Part model, mm, in its own coordinate system. A direction names the side the tool comes from. Round coordinates to 2 decimals unless told otherwise and drop trailing zeros. Order: outer loops, then holes, each group sorted by start corner. A loop starts at its lowest first (then second) coordinate and runs counter-clockwise, first axis right, second up. Notation, with made-up numbers: (80.25, 87.5) - (101.25, 87.5) arc R25 cw to (101.25, 105.5) - close; hole circle Ø1 at (7.5, 45). An arc over 180 degrees is marked (long way). Return JSON: item names as keys, results as strings. Group by question number.
Item 1: Saw through at B-B on z = 6. State how many separate pieces and enclosed holes the cut face has, and give its area (3 significant figures).
Item 2: Saw through at A-A on x = 10. List the corners of the cut face in (y, z), and give its area (3 significant figures).
Item 3: Drop flat-ended pins along their axis: pin 1 (3 mm diameter, centred on x = 46.25, z = 6, fed in from -Y); pin 2 (6 mm diameter, centred on x = 23, z = 3, fed in from +Y). Give the stop position or say it passes through.
Item 4: Saw through at C-C on y = 39. List the corners of the cut face in (x, z), and give its area (3 significant figures).
Item 5: Saw through at D-D on z = 10.25. List the corners of the cut face in (x, y), and give its area (3 significant figures).
Item 6: Probe probe 1 along X at (y, z) = (2.55, 6); probe 2 along X at (y, z) = (25.5, 9); probe 3 along Y at (x, z) = (57.6, 6). List the from-to ranges inside material, lowest first.
Item 7: Two-plate mould, pull along Y, no slides. Class faces 6 (the face through (32, 0, 6)), 7 (the face through (59.4, 54, 6)), 8 (the face through (32, 3, 0)), 9 (the face through (60, 59, 6)): released by +Y, released by -Y, zero draft, split by the parting line, or undercut.
Item 8: Tool access for faces 1 (the face through (58.18, 51.46, 6.56)), 2 (the face through (19.584, 1.726, 6.241)), 3 (the face through (64, 29, 6)), 4 (the face through (55, 47, 6)), 5 (the face through (9, 45, 6)): list every direction of +Z, -Z, +X, -X, +Y, -Y with a clear straight run to the whole face (end or side of a thin tool).
```python
from build123d import *

# Parameters (mm, degrees)
SKETCH1_W           = 64
SKETCH1_H           = 59
SKETCH1_W_2         = 50
SKETCH1_H_2         = 52
BOSS_EXTRUDE1_DEPTH = 12
SKETCH2_R           = 1.85
CUT_EXTRUDE1_DEPTH  = 10
SKETCH3_R           = 1.85
CUT_EXTRUDE2_DEPTH  = 10
SKETCH4_W           = 50
SKETCH4_H           = 12
SKETCH4_R           = 1.85
CUT_EXTRUDE4_DEPTH  = 10
SKETCH6_R           = 2.6
CUT_EXTRUDE5_DEPTH  = 2.4
SKETCH7_W           = 12
SKETCH7_H           = 2
BOSS_EXTRUDE2_DEPTH = 4


with BuildPart() as part:
    # Sketch1 → Boss-Extrude1 (new body)
    with BuildSketch(Plane.XY):
        with Locations((32, 29.5)):
            Rectangle(SKETCH1_W, SKETCH1_H)
        with Locations((32, 29.5)):
            Rectangle(SKETCH1_W_2, SKETCH1_H_2, mode=Mode.SUBTRACT)
    extrude(amount=BOSS_EXTRUDE1_DEPTH)

    # Sketch2 → Cut-Extrude1 (cut)
    with BuildSketch(Plane(origin=(0, 59, 0), x_dir=(1, 0, 0), z_dir=(0, 1, 0))):
        with Locations(Location((18, -9.7, 0), (0, 0, 180))):
            Circle(SKETCH2_R)
        with Locations(Location((46, -9.7, 0), (0, 0, 180))):
            Circle(SKETCH2_R)
        with Locations(Location((32, -9.7, 0), (0, 0, 180))):
            Circle(SKETCH2_R)
    extrude(amount=-CUT_EXTRUDE1_DEPTH, mode=Mode.SUBTRACT)

    # Sketch3 → Cut-Extrude2 (cut)
    with BuildSketch(Plane.XZ):
        with Locations(Location((17.75, 6, 0), (0, 0, 270))):
            Circle(SKETCH3_R)
        with Locations(Location((46.25, 6, 0), (0, 0, 180))):
            Circle(SKETCH3_R)
    extrude(amount=-CUT_EXTRUDE2_DEPTH, mode=Mode.SUBTRACT)

    # Sketch4 → Cut-Extrude4 (cut)
    with BuildSketch(Plane(origin=(0, 59, 0), x_dir=(1, 0, 0), z_dir=(0, 1, 0))):
        with Locations((32, -6)):
            Rectangle(SKETCH4_W, SKETCH4_H)
        with Locations((18, -9.7)):
            Circle(SKETCH4_R, mode=Mode.SUBTRACT)
        with Locations((32, -9.7)):
            Circle(SKETCH4_R, mode=Mode.SUBTRACT)
        with Locations((46, -9.7)):
            Circle(SKETCH4_R, mode=Mode.SUBTRACT)
    extrude(amount=-CUT_EXTRUDE4_DEPTH, mode=Mode.SUBTRACT)

    # Sketch6 → Cut-Extrude5 (cut)
    with BuildSketch(Plane(origin=(7, 0, 0), x_dir=(0, 0, -1), z_dir=(1, 0, 0))):
        with Locations((-6, 54)):
            Circle(SKETCH6_R)
    cut_extrude5 = extrude(amount=-CUT_EXTRUDE5_DEPTH, mode=Mode.SUBTRACT)

    # Mirror1: Cut-Extrude5 across plane
    add(cut_extrude5.mirror(Plane.ZY.offset(-32)), mode=Mode.SUBTRACT)

    # Sketch7 → Boss-Extrude2 (add)
    with BuildSketch(Plane.ZY.offset(-57)):
        with Locations((6, 46)):
            Rectangle(SKETCH7_W, SKETCH7_H)
    boss_extrude2 = extrude(amount=BOSS_EXTRUDE2_DEPTH)

    # Mirror2: Boss-Extrude2 across plane
    add(boss_extrude2.mirror(Plane.ZY.offset(-32)))


solid = part.part
```
Filled in:
{
 "1": {"separate pieces": "3", "enclosed holes": "0", "area": "966 mm^2"},
 "2": {"outline": "(0, 0) - (3.5, 0) - (3.5, 12) - (0, 12) - close; (45, 0) - (47, 0) - (47, 12) - (45, 12) - close", "area": "66.0 mm^2"},
 "3": {"pin 1": "passes through", "pin 2": "stops at y = 3.5"},
 "4": {"outline": "(0, 0) - (7, 0) - (7, 12) - (0, 12) - close; (57, 0) - (64, 0) - (64, 12) - (57, 12) - close", "area": "168 mm^2"},
 "5": {"outline": "(0, 0) - (64, 0) - (64, 59) - (57, 59) - (57, 47) - (53, 47) - (53, 45) - (57, 45) - (57, 3.5) - (7, 3.5) - (7, 45) - (11, 45) - (11, 47) - (7, 47) - (7, 59) - (0, 59) - close", "area": "1,020 mm^2"},
 "6": {"probe 1": "x = 0 to 15.9, 19.6 to 44.4, 48.1 to 64", "probe 2": "x = 0 to 7, 57 to 64", "probe 3": "y = 0 to 51.4, 56.6 to 59"},
 "7": {"face 6": "released by -Y", "face 7": "undercut", "face 8": "zero draft", "face 9": "released by +Y"},
 "8": {"face 1": "none", "face 2": "+Y, -Y", "face 3": "+Z, -Z, +X, +Y, -Y", "face 4": "+Z, -Z, +Y", "face 5": "+Z, -Z"}
}
